The drawing under review shows one solid part. Ordinate dimensions are in mm from its lowest x, y, z. Coordinates: 2 decimals unless noted, no trailing zeros. Loops run counter-clockwise (first coordinate to the right, second up) from the corner with the lowest first, then second, coordinate; pieces in that order, holes last. Notation, with made-up numbers: (38.5, 61.25) - (76.5, 61.25) arc R27 ccw to (76.5, 85.25) - close; hole circle Ø10 at (-6, 89). An arc over 180 degrees is marked (long way). Answer as a JSON object with one key per item and string values. Group by question number.
Item 1: Clearance check with a flat-ended pin moving along its axis: pin 1 (12 mm diameter, centred on x = 10.5, z = 62, fed in from -Y). State where the tip first meets the part, or that it passes through.
Item 2: Mouldability with a two-part tool opening along Z and no side actions: class the marked faces 1, 2, 3 and 4 as released by +Z, released by -Z, zero draft, split by the parting line, or undercut.
Item 3: We need section A-A (x = 29). Give the boundary of the cut face in (y, z).
Item 4: We need section B-B (z = 23). Give the boundary of the cut face in (x, y), then the cut area to 3 significant figures.
Item 5: We need section C-C (y = 2). Give the boundary of the cut face in (x, z), then the cut area to 4 significant figures.
Item 6: To check wall thickness, follow line 1 (Z direction, x = 17.5, y = 7) (1 decimal); line 2 (Z direction, x = 30, y = 6.25); line 3 (X direction, y = 7, z = 15). State the ranges of each line that lie inside material, in increasing order.
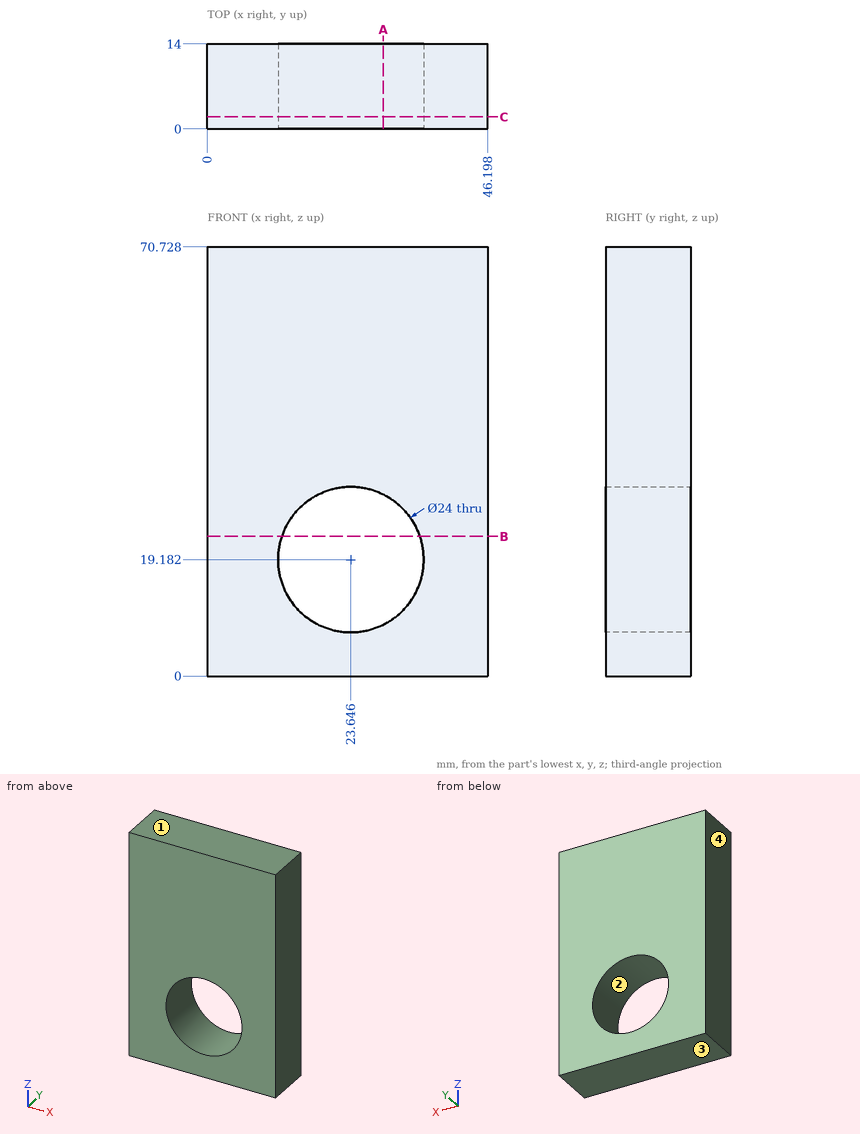
Check sheet entries:
{
 "1": {"pin 1": "stops at y = 0"},
 "2": {"face 1": "released by +Z", "face 2": "undercut", "face 3": "released by -Z", "face 4": "zero draft"},
 "3": {"outline": "(0, 0) - (14, 0) - (14, 8.44) - (0, 8.44) - close; (0, 29.92) - (14, 29.92) - (14, 70.73) - (0, 70.73) - close"},
 "4": {"outline": "(0, 0) - (12.27, 0) - (12.27, 14) - (0, 14) - close; (35.02, 0) - (46.2, 0) - (46.2, 14) - (35.02, 14) - close", "area": "328 mm2"},
 "5": {"outline": "(0, 0) - (46.2, 0) - (46.2, 70.73) - (0, 70.73) - close; hole circle Ø24 at (23.65, 19.18)", "area": "2,815 mm2"},
 "6": {"line 1": "z = 0 to 8.9, 29.5 to 70.7", "line 2": "z = 0 to 9, 29.36 to 70.73", "line 3": "x = 0 to 12.4, 34.89 to 46.2"}
}
